from build123d import *


# Not quite as in the source:
# - a fillet or chamfer that OpenCascade refuses, or shapes differently, is made with other operations: its cross-section is extruded or revolved along the edge and cut away or added


with BuildPart() as f1:
    # F0 (on Front) → F1 (revolve)
    with BuildSketch(Plane.XZ):
        Polygon((0, 2.4378150702), (0, 2.7715591714), (0, 9.970895946), (-2.0202985033, 9.970895946), (-2.0202985033, 8.6359195411), (-6.4543271437, 8.6359195411), (-6.4543271437, 9.9232187495), (-8.5521470755, 9.9232187495), (-8.5521470755, 7.0625548251), (-6.4543271437, 7.0625548251), (-6.4543271437, 4.7263461165), (-8.4091145545, 4.7263461165), (-8.4091145545, 2.4378150702), align=None)
    revolve(axis=Axis((0, 0, 6.3712275587), (0, 0, 1)))

    # F2: chamfer of 2.54 on 1 edges, made by hand


with BuildPart() as f2_tool2:
    # F2_s3 → F2_t4 (revolve)
    with BuildSketch(Plane.XZ):
        Polygon((-6.4543271437, 7.3832187495), (-8.9943271437, 9.9232187495), (-6.4543271437, 9.9232187495), align=None)
    revolve(axis=Axis((0, 0, 9.9232187495), (0, 0, 1)))

    split(bisect_by=Plane.XY.offset(8.6359195411), keep=Keep.TOP)


with BuildPart() as f1_1:
    add(f1.part)

    # F2_t1: cut F2_tool2
    add(f2_tool2.part, mode=Mode.SUBTRACT)


solid = f1_1.part
Could you check a few things on this model? Use its own coordinates, in mm. A direction names the side the tool comes from. Coordinates: 2 decimals unless noted, no trailing zeros. Loops run counter-clockwise (first coordinate to the right, second up) from the corner with the lowest first, then second, coordinate; pieces in that order, holes last.
1. Imagine slicing it at D-D (z = 7.5). Please give me the cut outline in (x, y), and give its area (3 significant figures).
2. Imagine slicing it at A-A (y = 0). Please give me the cut outline in (x, z), and give its area (3 significant figures).
3. For faces 1 (the face through (1.85, 8.35, 8.25)), 2 (the face through (2, 2, 8.636)), 3 (the face through (3, -6, 7.063)), which set-ups out of +Z, -Z, +X, -X, +Y, -Y let a thin tool reach every point of the face, with its end or its side?
4. For P1, Ø3, axis at y = 4, z = 8, coming from the -X side; P2, Ø4, axis at y = -2.5, z = 3, coming from the -X side; P3, Ø4, axis at x = 3.5, z = 5.5, coming from the -Y side, each with a flat end and sliding along its axis, tell me the tip position at first contact or that it passes through.
5. We'd pull the mould along X, two halves only. Please class faces 4 (the face through (0, 0, 9.971)), 5 (the face through (-8.02, -2.53, 3.57)), 6 (the face through (0.44, 1.97, 9.29)): released by +X, released by -X, zero draft, split by the parting line, or undercut.
6. Imagine slicing it at C-C (z = 4). Please give me the cut outline in (x, y).
7. I need wall thicknesses on L1, parallel to Z at x = -5.5, y = -3.75; L2, parallel to Y at x = -0.25, z = 4.25; L3, parallel to Z at x = -6.25, y = -4.75. Which ranges of each line are inside material? Lowest first, please.
Computed values:
1. outline: circle Ø17.1 at (0, 0)
1. area: 230 mm2
2. outline: (-8.55, 7.06) - (-6.45, 7.06) - (-6.45, 4.73) - (-8.41, 4.73) - (-8.41, 2.44) - (8.41, 2.44) - (8.41, 4.73) - (6.45, 4.73) - (6.45, 7.06) - (8.55, 7.06) - (8.55, 9.48) - (7.71, 8.64) - (2.02, 8.64) - (2.02, 9.97) - (-2.02, 9.97) - (-2.02, 8.64) - (-7.71, 8.64) - (-8.55, 9.48) - close
2. area: 102 mm2
3. face 1: +Z, -Z
3. face 2: +Z
3. face 3: none
4. P1: stops at x = -8.18
4. P2: stops at x = -8.39
4. P3: stops at y = -8.25
5. face 4: zero draft
5. face 5: split by the parting line
5. face 6: undercut
6. outline: circle Ø16.82 at (0, 0)
7. L1: z = 2.44 to 4.73, 7.06 to 8.64
7. L2: y = -8.41 to 8.41
7. L3: z = 2.44 to 4.73, 7.06 to 8.78
